Check sheet for the drawn part. Datum: minimum x, y, z corner. Units: mm. A direction names the side the tool comes from. Coordinates: 2 decimals unless noted, no trailing zeros. Order: outer loops, then holes, each group sorted by start corner. A loop starts at its lowest first (then second) coordinate and runs counter-clockwise, first axis right, second up.
1. Cross-section at C-C (y = 70). Enter the section's corners in (x, z) (3 decimals), then the cut area to 3 significant figures.
2. Thickness scan on line 1 (Y direction, x = 19.5, z = 48) (3 decimals); line 2 (Z direction, x = 42, y = 32) (3 decimals). Record the ranges inside material, lowest first.
3. Cross-section at A-A (z = 52). Enter the section's corners in (x, y) (3 decimals).
4. Set-up check for the marked faces 5 and 6: record each of +Z, -Z, +X, -X, +Y, -Y from which the full face is reachable in a straight line by a thin tool's end or side.
5. Draft check along Y on the marked faces 1, 2, 3 and 4. Enter one of: released by +Y, released by -Y, zero draft, split by the parting line, or undercut.
6. Gauge pin test, flat end, axial feed: pin 1 Ø23 at (x, y) = (53, 45.5) entering from +Z (3 decimals). Record the tip position at first contact, or that the pin passes through.
7. Cross-section at B-B (x = 67). Enter the section's corners in (y, z) (3 decimals).
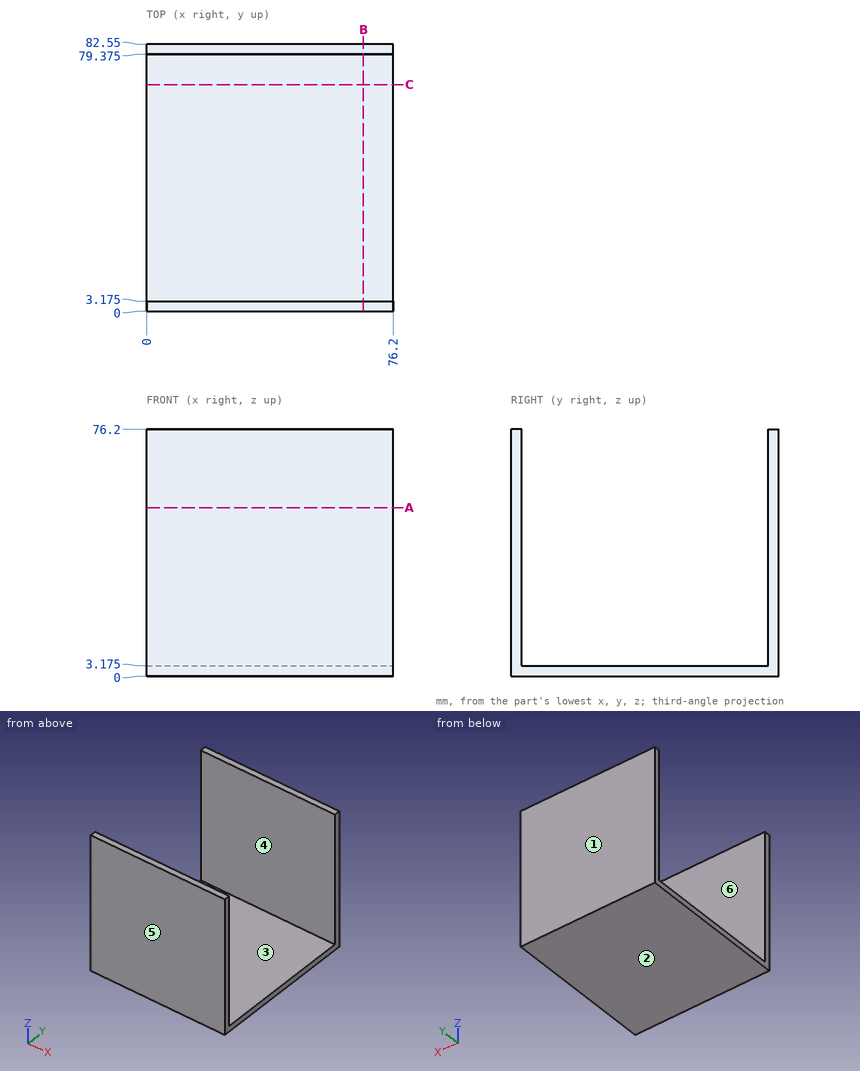
Data:
1. outline: (0, 0) - (76.2, 0) - (76.2, 3.175) - (0, 3.175) - close
1. area: 242 mm2
2. line 1: y = 0 to 3.175, 79.375 to 82.55
2. line 2: z = 0 to 3.175
3. outline: (0, 0) - (76.2, 0) - (76.2, 3.175) - (0, 3.175) - close; (0, 79.375) - (76.2, 79.375) - (76.2, 82.55) - (0, 82.55) - close
4. face 5: +Z, -Z, +X, -X, -Y
4. face 6: +Z, +X, -X
5. face 1: released by +Y
5. face 2: zero draft
5. face 3: undercut
5. face 4: undercut
6. pin 1: stops at z = 3.175
7. outline: (0, 0) - (82.55, 0) - (82.55, 76.2) - (79.375, 76.2) - (79.375, 3.175) - (3.175, 3.175) - (3.175, 76.2) - (0, 76.2) - close
